CAD build for the part. Positions are in the model's coordinates, mm. Face numbers are marked on the shaded views. A direction names the side the tool comes from. Coordinates: 2 decimals unless noted, no trailing zeros. Loops run counter-clockwise (first coordinate to the right, second up) from the corner with the lowest first, then second, coordinate; pieces in that order, holes last. Notation, with made-up numbers: (46.5, 13.5) -> (84.5, 13.5) arc R33 cw to (84.5, 52.5) -> close; hole circle Ø11 at (69, 54.25). An arc over 180 degrees is marked (long way). Answer as CSV lines item,"result". Start each with the question number.
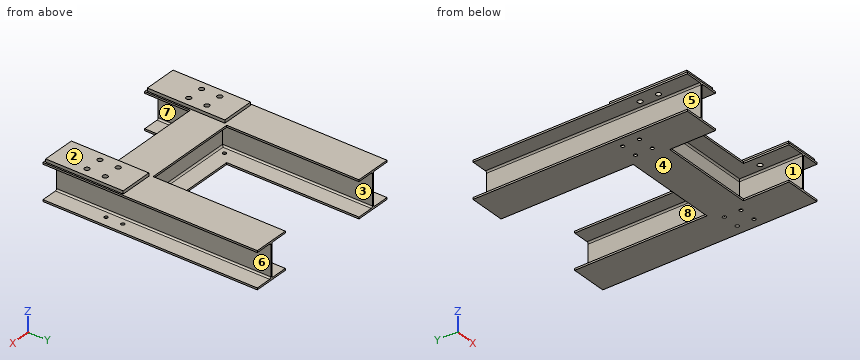
from build123d import *

# Parameters (mm, degrees)
F1_DEPTH  = 895.35
F2_W      = 279.4
F2_H      = 647.7
F3_DEPTH  = 25.4
F5_D      = 41.275
F5_DEPTH  = 76.2
F7_D      = 28.575
F7_DEPTH  = 76.2
F10_DEPTH = 552.45
F11_R     = 14.2875
F12_DEPTH = 76.2


with BuildPart() as f1:
    # F0 (on Front) → F1 (new body, symmetric)
    with BuildSketch(Plane.XZ):
        with BuildLine():
            Line((-400.05, 153.924), (-704.85, 153.924))
            Line((-704.85, 153.924), (-704.85, 138.684))
            Line((-704.85, 138.684), (-570.103, 138.684))
            ThreePointArc((-570.103, 138.684), (-561.122744, 134.964256), (-557.403, 125.984))
            Line((-557.403, 125.984), (-557.403, -125.984))
            ThreePointArc((-557.403, -125.984), (-561.122744, -134.964256), (-570.103, -138.684))
            Line((-570.103, -138.684), (-704.85, -138.684))
            Line((-704.85, -138.684), (-704.85, -153.924))
            Line((-704.85, -153.924), (-400.05, -153.924))
            Line((-400.05, -153.924), (-400.05, -138.684))
            Line((-400.05, -138.684), (-534.797, -138.684))
            ThreePointArc((-534.797, -138.684), (-543.777256, -134.964256), (-547.497, -125.984))
            Line((-547.497, -125.984), (-547.497, 125.984))
            ThreePointArc((-547.497, 125.984), (-543.777256, 134.964256), (-534.797, 138.684))
            Line((-534.797, 138.684), (-400.05, 138.684))
            Line((-400.05, 138.684), (-400.05, 153.924))
        make_face()
    extrude(amount=F1_DEPTH, both=True)

    # F2 (on face) → F3 (join)
    with BuildSketch(Plane.XY.offset(153.924)):
        with Locations((-552.45, -558.8)):
            Rectangle(F2_W, F2_H)
    extrude(amount=F3_DEPTH)

    # F5
    with Locations(Plane.XY.offset(179.324)):
        with Locations((-622.3, -438.15), (-482.6, -438.15), (-622.3, -590.55), (-482.6, -590.55)):
            Hole(F5_D / 2, depth=F5_DEPTH)

    # F7
    with Locations(Plane(origin=(0, 0, -153.924), x_dir=(1, 0, 0), z_dir=(0, 0, -1))):
        with Locations((-482.6, 431.8), (-482.6, 292.1), (-622.3, 431.8), (-622.3, 292.1)):
            Hole(F7_D / 2, depth=F7_DEPTH)



with BuildPart() as f8_1:
    # F8: instance of F1
    add(f1.part.mirror(Plane.YZ))


with BuildPart() as f1_1:
    add(f1.part)

    add(f8_1.part)  # F10 merges F8_1
    # F9 (on Right) → F10 (join, symmetric)
    with BuildSketch(Plane.YZ):
        with BuildLine():
            Line((-209.55, 153.924), (-514.35, 153.924))
            Line((-514.35, 153.924), (-514.35, 138.684))
            Line((-514.35, 138.684), (-379.603, 138.684))
            ThreePointArc((-379.603, 138.684), (-370.622744, 134.964256), (-366.903, 125.984))
            Line((-366.903, 125.984), (-366.903, -125.984))
            ThreePointArc((-366.903, -125.984), (-370.622744, -134.964256), (-379.603, -138.684))
            Line((-379.603, -138.684), (-514.35, -138.684))
            Line((-514.35, -138.684), (-514.35, -153.924))
            Line((-514.35, -153.924), (-209.55, -153.924))
            Line((-209.55, -153.924), (-209.55, -138.684))
            Line((-209.55, -138.684), (-344.297, -138.684))
            ThreePointArc((-344.297, -138.684), (-353.277256, -134.964256), (-356.997, -125.984))
            Line((-356.997, -125.984), (-356.997, 125.984))
            ThreePointArc((-356.997, 125.984), (-353.277256, 134.964256), (-344.297, 138.684))
            Line((-344.297, 138.684), (-209.55, 138.684))
            Line((-209.55, 138.684), (-209.55, 153.924))
        make_face()
    extrude(amount=F10_DEPTH, both=True)

    # F11 (on face) → F12 (cut)
    with BuildSketch(Plane(origin=(0, 0, -153.924), x_dir=(1, 0, 0), z_dir=(0, 0, -1))):
        with Locations((-482.6, 431.8)):
            Circle(F11_R)
        with Locations((-482.6, 292.1)):
            Circle(F11_R)
        with Locations((482.6, 431.8)):
            Circle(F11_R)
        with Locations((482.6, 292.1)):
            Circle(F11_R)
    extrude(amount=-F12_DEPTH, mode=Mode.SUBTRACT)


solid = f1_1.part
Item 1: Flat gauge pins, fed straight in: pin 1 Ø6 at (x, y) = (-224.5, -309.5) entering from +Z; pin 2 Ø4.5 at (x, z) = (-41, -149) entering from +Y; pin 3 Ø7.5 at (x, z) = (587, 161.5) entering from +Y; pin 4 Ø6 at (x, y) = (396.5, 311.5) entering from +Z. Where does each tip first touch, or does it go through?
Item 2: Saw through at C-C (x = -274). Write the cut outline in (y, z).
Item 3: Saw through at B-B (z = 36). Write the cut outline in (x, y).
Item 4: Two-plate mould, pull along Z, no slides. Class the marked faces 1, 2, 3 and 4: pulls with the +Z half, pulls with the -Z half, needs draft (parallel to the pull), parting line crosses it, or undercut.
Item 5: Wall check: probe 1 along Y at (x, z) = (-622.3, -150); probe 2 along Y at (x, z) = (622.3, 164); probe 3 along X at (y, z) = (-292.1, -145.5). Give the ranges that are in metal, low to high.
Item 6: Saw through at D-D (y = -590.55). Count the separate pieces of the cut face and the enclosed holes in it, plus the area to 3 significant figures.
Item 7: Which spindle directions (+Z, -Z, +X, -X, +Y, -Y) get a long thin tool onto all of the face, cutting with end or side? Do the marked faces 5, 6, 7 and 8. Say none if no direction does.
Geometry check:
1,pin 1,"z = 153.92"
1,pin 2,"y = -209.55"
1,pin 3,"y = -234.95"
1,pin 4,"through"
2,outline,"(-514.35, -153.92) -> (-209.55, -153.92) -> (-209.55, -138.68) -> (-344.3, -138.68) arc R12.7 cw to (-357, -125.98) -> (-357, 125.98) arc R12.7 cw to (-344.3, 138.68) -> (-209.55, 138.68) -> (-209.55, 153.92) -> (-514.35, 153.92) -> (-514.35, 138.68) -> (-379.6, 138.68) arc R12.7 cw to (-366.9, 125.98) -> (-366.9, -125.98) arc R12.7 cw to (-379.6, -138.68) -> (-514.35, -138.68) -> close"
3,outline,"(-557.4, -895.35) -> (-547.5, -895.35) -> (-547.5, -366.9) -> (547.5, -366.9) -> (547.5, -895.35) -> (557.4, -895.35) -> (557.4, 895.35) -> (547.5, 895.35) -> (547.5, -357) -> (-547.5, -357) -> (-547.5, 895.35) -> (-557.4, 895.35) -> close"
4,face 1,"undercut"
4,face 2,"pulls with the +Z half"
4,face 3,"undercut"
4,face 4,"pulls with the -Z half"
5,probe 1,"-895.35 to -446.09, -417.51 to -306.39, -277.81 to 895.35"
5,probe 2,"-882.65 to -611.19, -569.91 to -458.79, -417.51 to -234.95"
5,probe 3,"-704.85 to -636.59, -608.01 to -496.89, -468.31 to 468.31, 496.89 to 608.01, 636.59 to 704.85"
6,separate pieces,"6"
6,enclosed holes,"0"
6,area,"31,800 mm2"
7,face 5,"-X, +Y, -Y"
7,face 6,"+X, +Y, -Y"
7,face 7,"-Y"
7,face 8,"+Y"
